from build123d import *

# Parameters (mm, degrees)
SKIZZE1_W                       = 40
SKIZZE1_H                       = 40
AUFSATZ_LINEAR_AUSTRAGEN1_DEPTH = 6
VERRUNDUNG1_R                   = 5
SKIZZE2_W                       = 31.5
SKIZZE2_H                       = 31.5
SCHNITT_LINEAR_AUSTRAGEN1_DEPTH = 2.4
VERRUNDUNG2_R                   = 3
SKIZZE3_W                       = 26
SKIZZE3_H                       = 26
SCHNITT_LINEAR_AUSTRAGEN2_DEPTH = 2
VERRUNDUNG3_R                   = 2
SCHNITT_LINEAR_AUSTRAGEN3_REACH = 30.914
SKIZZE4_W                       = 4
SKIZZE4_H                       = 10.038850157


with BuildPart() as part:
    # Skizze1 → Aufsatz-Linear austragen1 (new body)
    with BuildSketch(Plane.XY):
        Rectangle(SKIZZE1_W, SKIZZE1_H)
    extrude(amount=AUFSATZ_LINEAR_AUSTRAGEN1_DEPTH)

    # Verrundung1
    verrundung1_edges = [part.edges().sort_by_distance(p)[0] for p in [
        (-20, 20, 3),
        (20, 20, 3),
        (20, -20, 3),
        (-20, -20, 3),
    ]]
    fillet(verrundung1_edges, radius=VERRUNDUNG1_R)

    # Skizze2 → Schnitt-Linear austragen1 (cut)
    with BuildSketch(Plane.XY.offset(6)):
        Rectangle(SKIZZE2_W, SKIZZE2_H)
    extrude(amount=-SCHNITT_LINEAR_AUSTRAGEN1_DEPTH, mode=Mode.SUBTRACT)

    # Verrundung2
    verrundung2_edges = [part.edges().sort_by_distance(p)[0] for p in [
        (-15.75, -15.75, 4.8),
        (-15.75, 15.75, 4.8),
        (15.75, 15.75, 4.8),
        (15.75, -15.75, 4.8),
    ]]
    fillet(verrundung2_edges, radius=VERRUNDUNG2_R)

    # Skizze3 → Schnitt-Linear austragen2 (cut)
    with BuildSketch(Plane.XY.offset(3.6)):
        Rectangle(SKIZZE3_W, SKIZZE3_H)
    extrude(amount=-SCHNITT_LINEAR_AUSTRAGEN2_DEPTH, mode=Mode.SUBTRACT)

    # Verrundung3
    verrundung3_edges = [part.edges().sort_by_distance(p)[0] for p in [
        (13, 13, 2.6),
        (13, -13, 2.6),
        (-13, -13, 2.6),
        (-13, 13, 2.6),
    ]]
    fillet(verrundung3_edges, radius=VERRUNDUNG3_R)

    # Schnitt-Linear austragen3: up to this face of the body (flat: up to its plane)
    schnitt_linear_austragen3_end = Plane(part.part.faces().sort_by_distance((0, 0, 1.6))[0])
    # Skizze4 → Schnitt-Linear austragen3 (cut, up to the picked face)
    with BuildSketch(Plane.XY.offset(6), mode=Mode.PRIVATE) as schnitt_linear_austragen3_sk1:
        with Locations((0, -17.296929977)):
            Rectangle(SKIZZE4_W, SKIZZE4_H)
    schnitt_linear_austragen3_tool1 = split(extrude(schnitt_linear_austragen3_sk1.sketch, amount=-SCHNITT_LINEAR_AUSTRAGEN3_REACH, mode=Mode.PRIVATE), bisect_by=schnitt_linear_austragen3_end, keep=Keep.BOTH, mode=Mode.PRIVATE)
    add(schnitt_linear_austragen3_tool1.solids().sort_by(Axis((0, -17.29693, 6), (0, 0, -1)))[0], mode=Mode.SUBTRACT)


solid = part.part
Work out the finished part from the listing and answer in its coordinate system (mm). A direction names the side the tool comes from. Give positions to 0.01 mm unless a question says otherwise; leave off trailing zeros. Order: outer loops, then holes, each group sorted by start corner. A loop starts at its lowest first (then second) coordinate and runs counter-clockwise, first axis right, second up. Notation, with made-up numbers: (-16.5, 5) -> (-7.5, 5) arc R22 ccw to (-7.5, 29) -> close; hole circle Ø9 at (45, 67). An arc over 180 degrees is marked (long way). Answer as a JSON object with one key per item and string values. Group by question number.
1. Consider line 1 along Y through (x, z) = (-9, 4.05); line 2 along X through (y, z) = (-0.5, 1.9). Determine where each line is inside the solid, lowest interval first. Write a range as [from, to].
2. The mould has two halves that part along X. Classify faces 1 (the flat face through (-20, 0, 3)), 2 (the cylindrical face through (19, 18, 3)), 3 (the flat face through (-15.75, 0, 5)): released by +X, released by -X, zero draft, split by the parting line, or undercut.
3. Section A-A on x = 1 is taken. Determine the outline of the cut face in (y, z).
4. Flat-ended cylindrical pins translate along their axes: pin 1 Ø3 at (x, y) = (2, 0.5) entering from +Z; pin 2 Ø1.9 at (x, z) = (0, 5) entering from -Y. Find the tip coordinate at first contact, or state that the pin passes through.
5. Section C-C on y = 2 is taken. Determine the outline of the cut face in (x, z), plus the area to 3 significant figures.
6. Section B-B on z = 4.45 is taken. Determine the outline of the cut face in (x, y), plus the area to 3 significant figures.
7. A tool of negligible diameter and unlimited length cuts with its end or side. For faces 4 (the flat face through (0, 20, 3)), 5 (the flat face through (2, -17, 4)), 6 (the cylindrical face through (12.43, 12.4, 2.59)), from which of +Z, -Z, +X, -X, +Y, -Y can it reach the whole face along a straight path? Write none if from no direction.
Result sheet:
{
 "1": {"line 1": "y = [-20, -15.75], [15.75, 20]", "line 2": "x = [-20, -13], [13, 20]"},
 "2": {"face 1": "released by -X", "face 2": "released by +X", "face 3": "undercut"},
 "3": {"outline": "(-20, 0) -> (20, 0) -> (20, 6) -> (15.75, 6) -> (15.75, 3.6) -> (13, 3.6) -> (13, 1.6) -> (-20, 1.6) -> close"},
 "4": {"pin 1": "stops at z = 1.6", "pin 2": "stops at y = 15.75"},
 "5": {"outline": "(-20, 0) -> (20, 0) -> (20, 6) -> (15.75, 6) -> (15.75, 3.6) -> (13, 3.6) -> (13, 1.6) -> (-13, 1.6) -> (-13, 3.6) -> (-15.75, 3.6) -> (-15.75, 6) -> (-20, 6) -> close", "area": "112 mm^2"},
 "6": {"outline": "(-20, -15) arc R5 ccw to (-15, -20) -> (-2, -20) -> (-2, -15.75) -> (-12.75, -15.75) arc R3 cw to (-15.75, -12.75) -> (-15.75, 12.75) arc R3 cw to (-12.75, 15.75) -> (12.75, 15.75) arc R3 cw to (15.75, 12.75) -> (15.75, -12.75) arc R3 cw to (12.75, -15.75) -> (2, -15.75) -> (2, -20) -> (15, -20) arc R5 ccw to (20, -15) -> (20, 15) arc R5 ccw to (15, 20) -> (-15, 20) arc R5 ccw to (-20, 15) -> close", "area": "577 mm^2"},
 "7": {"face 4": "+Z, -Z, +X, -X, +Y", "face 5": "+Z, -Y", "face 6": "+Z"}
}
